Here's how the part is built. I have some questions about the finished solid (model axes, mm). A direction names the side the tool comes from. Give positions to 0.01 mm unless a question says otherwise; leave off trailing zeros. Loops run counter-clockwise (first coordinate to the right, second up) from the corner with the lowest first, then second, coordinate; pieces in that order, holes last. Notation, with made-up numbers: (64.5, 35) - (91.5, 35) arc R15 ccw to (91.5, 43) - close; hole circle Ø8 at (52, 22). An arc over 180 degrees is marked (long way). Put each result on its own line as item: value. Start each with the question number.
Autodesk Inventor part; units mm, degrees
ref_plane "YZ Plane" through (0, 0, 0) normal (1, 0, 0) x (0, 1, 0)
ref_plane "XZ Plane" through (0, 0, 0) normal (0, 1, 0) x (-1, 0, 0)
ref_plane "XY Plane" through (0, 0, 0) normal (0, 0, 1) x (1, 0, 0)
sketch "CONTOURS" plane through (0, 0, 0) normal (0, 0, 1) x (1, 0, 0)
  arc A0 (354.6305, 1027.9401) -> (346.6305, 1027.9401) centre (350.6305, 1027.9401) ccw
  line L0 (346.6305, 1027.9401) -> (346.6305, 890.3591)
  arc A1 (56.6305, 596.8599) -> (346.6305, 890.3591) centre (-693.3695, 1627.9389) ccw
  line L1 (56.6305, 596.8599) -> (56.6305, 785.8598)
  line L2 (56.6305, 785.8598) -> (78.6305, 785.8598)
  arc A2 (78.6305, 785.8598) -> (86.6305, 785.8598) centre (82.6305, 785.8598) ccw
  line L3 (86.6305, 785.8598) -> (86.6305, 802.8598)
  arc A3 (86.6305, 802.8598) -> (78.6305, 802.8598) centre (82.6305, 802.8598) ccw
  line L4 (78.6305, 802.8598) -> (38.6305, 802.8598)
  line L5 (38.6305, 802.8598) -> (38.6305, 971.8598)
  line L6 (38.6305, 971.8598) -> (78.6305, 971.8598)
  arc A4 (78.6305, 971.8598) -> (86.6305, 971.8598) centre (82.6305, 971.8598) ccw
  line L7 (86.6305, 971.8598) -> (86.6305, 988.8598)
  arc A5 (86.6305, 988.8598) -> (78.6305, 988.8598) centre (82.6305, 988.8598) ccw
  line L8 (78.6305, 988.8598) -> (56.6305, 988.8598)
  line L9 (56.6305, 988.8598) -> (56.6305, 1177.8597)
  line L10 (56.6305, 1177.8597) -> (416.6305, 1177.8597)
  line L11 (416.6305, 1177.8597) -> (416.6305, 1155.9383)
  arc A6 (416.6305, 1155.9383) -> (416.6305, 1147.9383) centre (416.6305, 1151.9383) ccw
  line L12 (416.6305, 1147.9383) -> (434.6305, 1147.9383)
  line L13 (434.6305, 1147.9383) -> (434.6305, 1057.9383)
  line L14 (434.6305, 1057.9383) -> (416.6305, 1057.9383)
  arc A7 (416.6305, 1057.9383) -> (416.6305, 1049.9383) centre (416.6305, 1053.9383) ccw
  line L15 (416.6305, 1049.9383) -> (416.6305, 1027.9401)
  line L16 (416.6305, 1027.9401) -> (354.6305, 1027.9401)
sketch "LETTERS" plane through (0, 0, 0) normal (0, 0, 1) x (1, 0, 0)
  line L0 (214.8818, 1093.6309) -> (234.6305, 1102.9383)
  line L1 (234.6305, 1084.5494) -> (214.8818, 1093.6309)
  line L2 (214.8058, 1113.3691) -> (234.6305, 1113.3691)
  line L3 (217.3755, 1109.636) -> (214.8058, 1113.3691)
  line L4 (226.7124, 1099.1165) -> (226.7124, 1088.2213)
extrude "Extrusion1" add sketch "CONTOURS" along normal blind 18
properties part number "Support A1" material "Wood (Birch)"
1) I'm going to push flat-ended pins straight in: P1, Ø9, axis at y = 1043, z = 8, coming from the +X side; P2, Ø6, axis at y = 687.5, z = 4, coming from the -X side; P3, Ø5.5, axis at x = 428.5, z = 6.5, coming from the +Y side. Where does each tip first touch, or does it pass through?
2) Suppose I cut it at B-B on x = 395.5. Please give me the cut outline in (y, z).
3) I need wall thicknesses on line 1 (X direction, y = 1015, z = 4); line 2 (X direction, y = 1079, z = 14.5); line 3 (Y direction, x = 396, z = 16.5). Which ranges of each line are inside material? Lowest first, please.
4) Thinking about a two-plate mould opening in Y: for faces 1 (the flat face through (234, 1177.86, 9)), 2 (the flat face through (86.63, 794, 9)), 3 (the flat face through (386, 1027.94, 9)), 4 (the flat face through (190, 956, 0)), which applies, pulls with the +Y half, pulls with the -Y half, needs draft (parallel to the pull), parting line crosses it, or undercut?
5) Suppose I cut it at C-C on y = 1094.5. Please give me the cut outline in (x, z), plus the area to 3 significant figures.
6) Which directions (+Z, -Z, +X, -X, +Y, -Y) give clear straight access to the entire face, cutting with the end or side of a thin tool? Please do faces 5 (the flat face through (56.63, 1082, 9)), 6 (the flat face through (416.63, 1167, 9)), 7 (the flat face through (190, 956, 18)), 8 (the flat face through (59, 802.86, 9)), 9 (the flat face through (416.63, 1039, 9)).
7) Suppose I cut it at A-A on z = 4.75. Please give me the cut outline in (x, y).
Ans:
1. P1: stops at x = 416.63
1. P2: stops at x = 56.63
1. P3: stops at y = 1147.94
2. outline: (1027.94, 0) - (1177.86, 0) - (1177.86, 18) - (1027.94, 18) - close
3. line 1: x = 56.63 to 346.63
3. line 2: x = 56.63 to 434.63
3. line 3: y = 1027.94 to 1177.86
4. face 1: pulls with the +Y half
4. face 2: undercut
4. face 3: pulls with the -Y half
4. face 4: needs draft
5. outline: (56.63, 0) - (434.63, 0) - (434.63, 18) - (56.63, 18) - close
5. area: 6,800 mm²
6. face 5: +Z, -Z, -X, +Y
6. face 6: +Z, -Z, +X, +Y
6. face 7: +Z, +X, -X, +Y, -Y
6. face 8: +Z, -Z, -X
6. face 9: +Z, -Z, +X, -Y
7. outline: (38.63, 802.86) - (78.63, 802.86) arc R4 cw to (86.63, 802.86) - (86.63, 785.86) arc R4 cw to (78.63, 785.86) - (56.63, 785.86) - (56.63, 596.86) arc R1275 ccw to (346.63, 890.36) - (346.63, 1027.94) arc R4 cw to (354.63, 1027.94) - (416.63, 1027.94) - (416.63, 1049.94) arc R4 cw to (416.63, 1057.94) - (434.63, 1057.94) - (434.63, 1147.94) - (416.63, 1147.94) arc R4 cw to (416.63, 1155.94) - (416.63, 1177.86) - (56.63, 1177.86) - (56.63, 988.86) - (78.63, 988.86) arc R4 cw to (86.63, 988.86) - (86.63, 971.86) arc R4 cw to (78.63, 971.86) - (38.63, 971.86) - close
